Autodesk Inventor part; units mm, degrees
ref_plane "YZ Plane" through (0, 0, 0) normal (1, 0, 0) x (0, 1, 0)
ref_plane "XZ Plane" through (0, 0, 0) normal (0, 1, 0) x (-1, 0, 0)
ref_plane "XY Plane" through (0, 0, 0) normal (0, 0, 1) x (1, 0, 0)
sketch "スケッチ1" plane through (0, 0, 0) normal (0, 0, 1) x (1, 0, 0)
  line L0 (0, 0) -> (3, 0)
  line L1 (3, 0) -> (3, -15)
  line L2 (3, -15) -> (0, -15)
  line L3 (0, -15) -> (0, 0)
  line L4 (-9, 0) -> (-6, 0)
  line L5 (-6, 0) -> (-6, -15)
  line L6 (-6, -15) -> (-9, -15)
  line L7 (-9, -15) -> (-9, 0)
  line L8 (0, -30) -> (3, -30)
  line L9 (3, -30) -> (3, -45)
  line L10 (3, -45) -> (0, -45)
  line L11 (0, -45) -> (0, -30)
  line L12 (-9, -30) -> (-6, -30)
  line L13 (-6, -30) -> (-6, -45)
  line L14 (-6, -45) -> (-9, -45)
  line L15 (-9, -45) -> (-9, -30)
  line L16 (-87.5, 3) -> (81.5, 3)
  line L17 (-87.5, 3) -> (-87.5, -48)
  line L18 (-87.5, -48) -> (81.5, -48)
  line L19 (81.5, -48) -> (81.5, 3)
  circle A0 centre (-83, -1.5) radius 1.5
  circle A1 centre (77, -1.5) radius 1.5
  circle A2 centre (77, -43.5) radius 1.5
  circle A3 centre (-83, -43.5) radius 1.5
  circle A4 centre (3, -1.05) radius 1.05
  circle A5 centre (3, -13.95) radius 1.05
  circle A6 centre (0, -13.95) radius 1.05
  circle A7 centre (0, -1.05) radius 1.05
  circle A8 centre (-6, -1.05) radius 1.05
  circle A9 centre (-6, -13.95) radius 1.05
  circle A10 centre (-9, -13.95) radius 1.05
  circle A11 centre (-9, -1.05) radius 1.05
  circle A12 centre (-6, -31.05) radius 1.05
  circle A13 centre (-6, -43.95) radius 1.05
  circle A14 centre (-9, -43.95) radius 1.05
  circle A15 centre (-9, -31.05) radius 1.05
  circle A16 centre (0, -31.05) radius 1.05
  circle A17 centre (3, -31.05) radius 1.05
  circle A18 centre (3, -43.95) radius 1.05
  circle A19 centre (0, -43.95) radius 1.05
  circle A20 centre (-13.5, -7.5) radius 1.5
  circle A21 centre (7.5, -7.5) radius 1.5
  circle A22 centre (7.5, -37.5) radius 1.5
  circle A23 centre (-13.5, -37.5) radius 1.5
  line L20 (45, -30) -> (45, -45)
  line L21 (45, -45) -> (42, -45)
  circle A24 centre (42, -43.95) radius 1.05
  line L22 (42, -45) -> (42, -30)
  circle A25 centre (45, -43.95) radius 1.05
  line L23 (42, 0) -> (45, 0)
  line L24 (45, 0) -> (45, -15)
  line L25 (45, -15) -> (42, -15)
  line L26 (42, -15) -> (42, 0)
  circle A26 centre (45, -1.05) radius 1.05
  circle A27 centre (42, -1.05) radius 1.05
  circle A28 centre (42, -13.95) radius 1.05
  circle A29 centre (45, -13.95) radius 1.05
  line L27 (42, -30) -> (45, -30)
  circle A30 centre (45, -31.05) radius 1.05
  circle A31 centre (42, -31.05) radius 1.05
  circle A32 centre (49.5, -37.5) radius 1.5
  circle A33 centre (49.5, -7.5) radius 1.5
  line L28 (-51, -15) -> (-51, 0)
  line L29 (-48, -30) -> (-48, -45)
  line L30 (-51, -45) -> (-51, -30)
  line L31 (-48, 0) -> (-48, -15)
  circle A34 centre (-48, -31.05) radius 1.05
  circle A35 centre (-48, -43.95) radius 1.05
  circle A36 centre (-51, -13.95) radius 1.05
  circle A37 centre (-55.5, -7.5) radius 1.5
  circle A38 centre (-48, -1.05) radius 1.05
  circle A39 centre (-51, -1.05) radius 1.05
  circle A40 centre (-48, -13.95) radius 1.05
  line L32 (-48, -45) -> (-51, -45)
  line L33 (-51, -30) -> (-48, -30)
  line L34 (-51, 0) -> (-48, 0)
  line L35 (-48, -15) -> (-51, -15)
  circle A41 centre (-51, -43.95) radius 1.05
  circle A42 centre (-51, -31.05) radius 1.05
  circle A43 centre (-55.5, -37.5) radius 1.5
  point P0 (0, -42.9)
  point P1 (0, -32.1)
  point P2 (3, -32.1)
  point P3 (3, -42.9)
  point P4 (0, -2.1)
  point P5 (3, -2.1)
  point P6 (3, -12.9)
  point P7 (0, -12.9)
  point P8 (-9, -2.1)
  point P9 (-6, 0)
  point P10 (-6, -2.1)
  point P11 (-6, -12.9)
  point P12 (-9, -12.9)
  point P13 (-9, -32.1)
  point P14 (-6, -32.1)
  point P15 (-6, -42.9)
  point P16 (-9, -42.9)
  point P17 (-4.9275, 0)
  point P18 (1, -30)
  point P19 (-51, -32.1)
  point P20 (-48, -32.1)
  point P21 (-48, -42.9)
  point P22 (-51, -42.9)
  point P23 (42, -12.9)
  point P24 (42, -2.1)
  point P25 (45, -2.1)
  point P26 (45, -12.9)
  point P27 (42, -32.1)
  point P28 (45, -32.1)
  point P29 (45, -42.9)
  point P30 (42, -42.9)
  point P31 (-51, -12.9)
  point P32 (-51, -2.1)
  point P33 (-51, 0)
  point P34 (-48, -2.1)
  point P35 (-48, -12.9)
  dimension "d0" = 3
  dimension "d1" = 15
  dimension "d2" = 3
  dimension "d3" = 15
  dimension "d4" = 3
  dimension "d5" = 15
  dimension "d6" = 3
  dimension "d7" = 15
  dimension "d8" = 15
  dimension "d9" = 6
  dimension "d10" = 3
  dimension "d11" = 3
  dimension "d12" = 3
  dimension "d13" = 3
  dimension "d14" = 3
  dimension "d15" = 3
  dimension "d16" = 4.5
  dimension "d17" = 4.5
  dimension "d18" = 4.5
  dimension "d19" = 4.5
  dimension "d20" = 4.5
  dimension "d21" = 4.5
  dimension "d22" = 4.5
  dimension "d23" = 4.5
  dimension "d24" = 160
  dimension "d25" = 74
  dimension "d26" = 2.1
  dimension "d27" = 3
  dimension "d28" = 3
  dimension "d29" = 3
  dimension "d30" = 3
  dimension "d31" = 4.5
  dimension "d32" = 4.5
  dimension "d33" = 4.5
  dimension "d34" = 4.5
  dimension "d35" = 7.5
  dimension "d36" = 7.5
  dimension "d37" = 7.5
  dimension "d38" = 7.5
  dimension "d39" = 3
  dimension "d40" = 15
  dimension "d41" = 3
  dimension "d42" = 15
  dimension "d43" = 15
  dimension "d44" = 2.1
  dimension "d45" = 3
  dimension "d46" = 3
  dimension "d47" = 4.5
  dimension "d48" = 4.5
  dimension "d49" = 7.5
  dimension "d50" = 7.5
  dimension "d51" = 3
  dimension "d52" = 15
  dimension "d53" = 3
  dimension "d54" = 15
  dimension "d55" = 3
  dimension "d56" = 3
  dimension "d57" = 4.5
  dimension "d58" = 4.5
  dimension "d59" = 7.5
  dimension "d60" = 7.5
  dimension "d61" = 3
  dimension "d62" = 90
  dimension "d63" = 36.5
sketch "スケッチ2" plane through (0, 0, 0) normal (0, 0, 1) x (1, 0, 0)
  circle A0 centre (-83, -1.5) radius 1.5
  circle A1 centre (-83, -43.5) radius 1.5
  circle A2 centre (-55.5, -7.5) radius 1.5
  circle A3 centre (-55.5, -37.5) radius 1.5
  circle A4 centre (-13.5, -37.5) radius 1.5
  circle A5 centre (-13.5, -7.5) radius 1.5
  circle A6 centre (7.5, -7.5) radius 1.5
  circle A7 centre (7.5, -37.5) radius 1.5
  circle A8 centre (49.5, -37.5) radius 1.5
  circle A9 centre (49.5, -7.5) radius 1.5
  circle A10 centre (77, -1.5) radius 1.5
  circle A11 centre (77, -43.5) radius 1.5
  line L0 (-87.5, 3) -> (81.5, 3)
  line L1 (-87.5, 3) -> (-87.5, -52.3382)
  line L2 (81.5, 3) -> (81.5, -52.3382)
  line L3 (-43, -297) -> (37, -297)
  line L4 (-43, -297) -> (-163, -142.321)
  line L5 (37, -297) -> (157, -142.321)
  line L6 (157, -142.321) -> (157, -92.4008)
  line L7 (-163, -142.321) -> (-163, -92.4008)
  arc A12 (-163, -92.4008) -> (-87.5, -52.3382) centre (-157.9321, -10.7785) ccw
  arc A13 (81.5, -52.3382) -> (157, -92.4008) centre (151.9321, -10.7785) ccw
  point P0 (0, 0)
  dimension "d66" = 80
  dimension "d67" = 300
  dimension "d68" = 44.5
  dimension "d69" = 44.5
  dimension "d70" = 320
  dimension "d71" = 75.5
  dimension "d72" = 75.5
extrude "押し出し1" add sketch "スケッチ2" along normal blind 1.5
sketch "スケッチ3" plane through (0, 0, 1.5) normal (0, 0, 1) x (1, 0, 0)
  arc A0 (81.5, -62.77) -> (157, -104.1946) centre (152.6935, -22.5286) ccw
  line L0 (81.5, -62.77) -> (81.5, 3)
  line L1 (81.5, 3) -> (-87.5, 3)
  line L2 (-87.5, 3) -> (-87.5, -62.77)
  arc A1 (-163, -104.1946) -> (-87.5, -62.77) centre (-158.6935, -22.5286) ccw
  line L3 (-163, -104.1946) -> (-163, -142.321)
  line L4 (-163, -142.321) -> (-43, -297)
  line L5 (-43, -297) -> (37, -297)
  line L6 (37, -297) -> (157, -142.321)
  line L7 (157, -142.321) -> (157, -104.1946)
  circle A2 centre (77, -43.5) radius 1.5
  circle A3 centre (49.5, -7.5) radius 1.5
  circle A4 centre (7.5, -37.5) radius 1.5
  circle A5 centre (7.5, -7.5) radius 1.5
  circle A6 centre (-13.5, -7.5) radius 1.5
  circle A7 centre (-13.5, -37.5) radius 1.5
  circle A8 centre (-55.5, -37.5) radius 1.5
  circle A9 centre (-55.5, -7.5) radius 1.5
  circle A10 centre (-83, -43.5) radius 1.5
  circle A11 centre (-83, -1.5) radius 1.5
  circle A12 centre (49.5, -37.5) radius 1.5
  circle A13 centre (77, -1.5) radius 1.5
  line L8 (81.5, 3) -> (-87.5, 3)
  line L9 (-87.5, 3) -> (-57.4301, 94.7393)
  line L10 (-57.4301, 94.7393) -> (-30.5041, 94.7393)
  line L11 (-30.5041, 94.7393) -> (-30.5041, 42.9458)
  line L12 (-30.5041, 42.9458) -> (24.5041, 42.9458)
  line L13 (24.5041, 42.9458) -> (24.5041, 94.7393)
  line L14 (24.5041, 94.7393) -> (51.4301, 94.7393)
  line L15 (51.4301, 94.7393) -> (81.5, 3)
  point P0 (0, 0)
  dimension "d75" = 56.9959
  dimension "d76" = 56.9959
equation "\"d69\" = d68"
equation "\"d72\" = d71"
equation "\"d76\" = d75"
properties part number "シールド" material "ポリカーボネート、クリア"
For this review, take the finished solid that the model builds, in its own axes (mm). Round coordinates to 2 decimals unless told otherwise and drop trailing zeros. Loops run counter-clockwise (first coordinate to the right, second up) from the corner with the lowest first, then second, coordinate; pieces in that order, holes last. Notation, with made-up numbers: (79.25, 53.25) - (127.25, 53.25) arc R22 cw to (127.25, 75.25) - close; hole circle Ø8 at (-8.75, -12). An arc over 180 degrees is marked (long way). Use one line per item in the form item = value.
1) We need section A-A on z = 1. State how many separate pieces and enclosed holes the cut face has, then the cut area to 3 significant figures.
Solutions:
separate_pieces = 1
enclosed_holes = 12
area = 64,600 mm2
2) Wall thickness on probe 1 along Y at (x, z) = (-13.5, 1.15); probe 2 along Y at (x, z) = (77, 0.8); probe 3 along X at (y, z) = (-20.5, 0.25): over which ranges is each line inside the solid? List them lowest first.
Solutions:
probe_1 = -297 to -39, -36 to -9, -6 to 3
probe_2 = -245.44 to -45, -42 to -3, 0 to 3
probe_3 = -87.5 to 81.5
3) Clearance check with flat-ended pins moving along their axes: P1, Ø0.8, axis at y = -28, z = 1, coming from the +X side; P2, Ø2.5, axis at x = -13.5, y = -37.5, coming from the -Z side. State where each tip first meets the part, or that it passes through.
Solutions:
P1 = 81.5
P2 = through
4) We need section C-C on y = -223. Write out the cut boundary in (x, z), then the cut area to 3 significant figures.
Solutions:
outline = (-100.41, 0) - (94.41, 0) - (94.41, 1.5) - (-100.41, 1.5) - close
area = 292 mm2
5) We need section B-B on x = 131. Write out the cut boundary in (y, z).
Solutions:
outline = (-175.83, 0) - (-89.83, 0) - (-89.83, 1.5) - (-175.83, 1.5) - close
